Geometry check sheet. Reference: the model listing, model coordinates, mm. A direction names the side the tool comes from. Coordinates: 2 decimals unless noted, no trailing zeros. Order: outer loops, then holes, each group sorted by start corner. A loop starts at its lowest first (then second) coordinate and runs counter-clockwise, first axis right, second up. Notation, with made-up numbers: (-37, 69.25) - (-7, 69.25) arc R22 cw to (-7, 91.25) - close; hole circle Ø10 at (-25, 25.25). An arc over 180 degrees is marked (long way). Use CSV: the item, a comma, the result in double quotes. Start each with the question number.
1) Thickness scan on probe 1 along X at (y, z) = (0, 3.55); probe 2 along X at (y, z) = (3, 0.25); probe 3 along Z at (x, y) = (38, 15). Record the ranges inside material, lowest first. Write a range as [from, to].
2) Draft check along X on faces 3 (the flat face through (55, 0, 0)), 4 (the cylindrical face through (27, 12, 0)), 5 (the cylindrical face through (44.81, -0.96, -2.46)). Enter one of: released by +X, released by -X, zero draft, split by the parting line, or undercut.
3) Depth check by flat-ended pin: P1, Ø6.5, axis at x = 10, y = 0, coming from the +Z side; P2, Ø3, axis at y = 14.5, z = -1, coming from the +X side. Enter the tip coordinate at first touch or a pass-through.
4) Tool access check on faces 1 (the flat face through (12, -2, 0)), 2 (the flat face through (0, 0, 0)). Record the directions out of +Z, -Z, +X, -X, +Y, -Y that give a thin tool (end or side, any length) a straight path to the whole face; none if there is none.
5) Sectioned sample at D-D, the plane z = -4. Record the cut outline in (x, y), and give its area (3 significant figures).
6) Sectioned sample at C-C, the plane x = 50. Record the cut outline in (y, z).
7) Sectioned sample at A-A, the plane x = 42.5. Record the cut outline in (y, z).
8) Sectioned sample at B-B, the plane y = -15. Record the cut outline in (x, z), and give its area (3 significant figures).
Solid Edge part; units mm, degrees
sketch "Sketch1" plane through (0, 0, 0) normal (1, 0, 0) x (0, 1, 0)
  circle A0 centre (-15, 0) radius 3
  circle A1 centre (15, 0) radius 3
  line L0 (20, -5) -> (-20, -5)
  line L1 (-20, -5) -> (-20, 5)
  line L2 (-20, 5) -> (20, 5)
  line L3 (20, 5) -> (20, -5)
  dimension "D1" = 20
  dimension "D2" = 20
extrude "Protrusion1" add sketch "Sketch1" along normal blind 50
sketch "Sketch2" plane through (25, 0, 5) normal (0, 0, 1) x (1, 0, 0)
  circle A0 centre (17.5, 0) radius 2.5
  circle A1 centre (-15, 0) radius 2.5
extrude "Cutout1" cut sketch "Sketch2" against normal up to next
sketch "Sketch3" plane through (50, 0, 0) normal (1, 0, 0) x (0, 1, 0)
  line L0 (-20, -5) -> (20, -5)
  line L1 (20, -5) -> (20, 5)
  line L2 (20, 5) -> (-20, 5)
  line L3 (-20, 5) -> (-20, -5)
  circle A0 centre (15, 0) radius 3
  circle A1 centre (-15, 0) radius 3
extrude "ExtrudedProtrusion_4" add sketch "Sketch3" along normal blind 5
fillet "Round_1" radius 3 2 edges at (27.5, -20, -5) (27.5, 20, -5)
sketch "Sketch4" plane through (27.5, 0, 5) normal (0, 0, 1) x (0, -1, 0)
  circle A0 centre (0, -17.5) radius 4.25
  circle A1 centre (0, 15) radius 4.25
extrude "ExtrudedCutout_2" cut sketch "Sketch4" against normal blind 5
properties material "ABS Plastic, high impact"
Evaluation:
1,probe 1,"[0, 5.75], [14.25, 38.25], [46.75, 55]"
1,probe 2,"[0, 6.99], [13.01, 39.49], [45.51, 55]"
1,probe 3,"[-5, -3], [3, 5]"
2,face 3,"released by +X"
2,face 4,"zero draft"
2,face 5,"undercut"
3,P1,"z = 0"
3,P2,"through"
4,face 1,"+Z"
4,face 2,"+Z, -Z, -X, +Y, -Y"
5,outline,"(0, -19.24) - (55, -19.24) - (55, 19.24) - (0, 19.24) - close; hole circle Ø5 at (10, 0); hole circle Ø5 at (42.5, 0)"
5,area,"2,080 mm²"
6,outline,"(-20, -2) arc R3 ccw to (-17, -5) - (17, -5) arc R3 ccw to (20, -2) - (20, 5) - (-20, 5) - close; hole circle Ø6 at (-15, 0); hole circle Ø6 at (15, 0)"
7,outline,"(-20, -2) arc R3 ccw to (-17, -5) - (-2.5, -5) - (-2.5, 0) - (-4.25, 0) - (-4.25, 5) - (-20, 5) - close; (2.5, -5) - (17, -5) arc R3 ccw to (20, -2) - (20, 5) - (4.25, 5) - (4.25, 0) - (2.5, 0) - close; hole circle Ø6 at (-15, 0); hole circle Ø6 at (15, 0)"
8,outline,"(0, -5) - (55, -5) - (55, -3) - (0, -3) - close; (0, 3) - (55, 3) - (55, 5) - (0, 5) - close"
8,area,"220 mm²"
